Build history of the part. All positions in model axes, mm. A direction names the side the tool comes from. Give positions to 0.01 mm unless a question says otherwise; leave off trailing zeros. Write each loop counter-clockwise with the first axis right and the second up, starting at its lowest first coordinate (ties: lowest second). Pieces come first, ordered by that corner, then holes.
from build123d import *

# Parameters (mm, degrees)
SKETCH_1_W           = 85
SKETCH_1_H           = 65
EXTRUDE_1_DEPTH      = 10
CUT_EXTRUDE_1_REACH  = 109.471
SKETCH_2_R           = 1.7
CUT_EXTRUDE_2_REACH  = 109.471
SKETCH_3_W           = 85
SKETCH_3_H           = 65
CUT_EXTRUDE_4_REACH  = 102.464
CUT_EXTRUDE_7_DEPTH  = 6
SKETCH_6_W           = 4
SKETCH_6_H           = 16
CUT_EXTRUDE_8_DEPTH  = 6
CUT_EXTRUDE_11_DEPTH = 2
SKETCH_15_W          = 14
SKETCH_15_H          = 4.4
CUT_EXTRUDE_13_DEPTH = 8
CHAMFER_1_SIZE       = 1


with BuildPart() as part:
    # 草图1 → 凸台-拉伸1 (new body)
    with BuildSketch(Plane.XY):
        with Locations((42.5, 32.5)):
            Rectangle(SKETCH_1_W, SKETCH_1_H)
    extrude(amount=EXTRUDE_1_DEPTH)

    # 草图2 → 切除-拉伸1 (cut, up to next)
    with BuildSketch(Plane(origin=(0, 0, 0), x_dir=(-1, 0, 0), z_dir=(0, 0, -1)), mode=Mode.PRIVATE) as cut_extrude_1_sk1:
        with Locations((-76.166921514, 56.442524765)):
            Circle(SKETCH_2_R)
    cut_extrude_1_tool1 = extrude(cut_extrude_1_sk1.sketch, amount=-CUT_EXTRUDE_1_REACH, mode=Mode.PRIVATE) & part.part
    # 草图2 → 切除-拉伸1 (cut, up to next)
    with BuildSketch(Plane(origin=(0, 0, 0), x_dir=(-1, 0, 0), z_dir=(0, 0, -1)), mode=Mode.PRIVATE) as cut_extrude_1_sk2:
        with Locations((-8.888803658, 56.442524765)):
            Circle(SKETCH_2_R)
    cut_extrude_1_tool2 = extrude(cut_extrude_1_sk2.sketch, amount=-CUT_EXTRUDE_1_REACH, mode=Mode.PRIVATE) & part.part
    # 草图2 → 切除-拉伸1 (cut, up to next)
    with BuildSketch(Plane(origin=(0, 0, 0), x_dir=(-1, 0, 0), z_dir=(0, 0, -1)), mode=Mode.PRIVATE) as cut_extrude_1_sk3:
        with Locations((-76.166921514, 8.41508509)):
            Circle(SKETCH_2_R)
    cut_extrude_1_tool3 = extrude(cut_extrude_1_sk3.sketch, amount=-CUT_EXTRUDE_1_REACH, mode=Mode.PRIVATE) & part.part
    # 草图2 → 切除-拉伸1 (cut, up to next)
    with BuildSketch(Plane(origin=(0, 0, 0), x_dir=(-1, 0, 0), z_dir=(0, 0, -1)), mode=Mode.PRIVATE) as cut_extrude_1_sk4:
        with Locations((-8.888803658, 8.41508509)):
            Circle(SKETCH_2_R)
    cut_extrude_1_tool4 = extrude(cut_extrude_1_sk4.sketch, amount=-CUT_EXTRUDE_1_REACH, mode=Mode.PRIVATE) & part.part
    add(cut_extrude_1_tool1.solids().sort_by_distance((76.166922, 56.442525, 0))[0], mode=Mode.SUBTRACT)
    add(cut_extrude_1_tool2.solids().sort_by_distance((8.888804, 56.442525, 0))[0], mode=Mode.SUBTRACT)
    add(cut_extrude_1_tool3.solids().sort_by_distance((76.166922, 8.415085, 0))[0], mode=Mode.SUBTRACT)
    add(cut_extrude_1_tool4.solids().sort_by_distance((8.888804, 8.415085, 0))[0], mode=Mode.SUBTRACT)

    # 草图3 → 切除-拉伸2 (cut, up to next)
    with BuildSketch(Plane(origin=(0, 0, 0), x_dir=(-1, 0, 0), z_dir=(0, 0, -1)), mode=Mode.PRIVATE) as cut_extrude_2_sk1:
        with Locations((-42.5, 32.5)):
            Rectangle(SKETCH_3_W, SKETCH_3_H)
        Polygon((-5, 33.462892894), (-5.871324699, 34.334217592), (-5.87504445, 53.137061214), (-5, 54.017366187), (-5, 57.982143592), (-6.992565577, 59.974709169), (-23.773560915, 59.974709169), (-24.394872914, 59.353397171), (-54.61482093, 59.349677419), (-55.245113202, 59.974709169), (-77.982184232, 59.974709169), (-79.974749809, 57.982143592), (-79.97474981, 54.295829484), (-78.032030648, 52.353110322), (-78.028310897, 12.45999492), (-79.97474981, 10.508295484), (-79.97474981, 6.992565577), (-77.982184232, 5), (-74.414239441, 5), (-73.152434681, 6.26180476), (-60.043505207, 6.265524511), (-58.772720173, 5), (-32.926479725, 5), (-31.743585303, 6.182894422), (-17.461559563, 6.186614173), (-16.269684867, 5), (-6.992565577, 5), (-5, 6.992565577), align=None, mode=Mode.SUBTRACT)
    cut_extrude_2_tool1 = extrude(cut_extrude_2_sk1.sketch, amount=-CUT_EXTRUDE_2_REACH, mode=Mode.PRIVATE) & part.part
    add(cut_extrude_2_tool1.solids().sort_by_distance((42.5, 63.929953, 0))[0], mode=Mode.SUBTRACT)

    # 草图4 → 切除-拉伸4 (cut, up to next)
    with BuildSketch(Plane(origin=(0, 0, 0), x_dir=(-1, 0, 0), z_dir=(0, 0, -1)), mode=Mode.PRIVATE) as cut_extrude_4_sk1:
        Polygon((-73.152434681, 6.26180476), (-73.152434681, 20.032317315), (-69.831576581, 23.353175415), (-46.787984184, 23.353175415), (-20.851296271, 23.353175415), (-17.461559563, 19.963438707), (-17.461559563, 6.186614173), (-17.461559563, 0.193960815), (-73.152434681, 0.193960815), align=None)
    cut_extrude_4_tool1 = extrude(cut_extrude_4_sk1.sketch, amount=-CUT_EXTRUDE_4_REACH, mode=Mode.PRIVATE) & part.part
    add(cut_extrude_4_tool1.solids().sort_by_distance((45.311727, 11.681443, 0))[0], mode=Mode.SUBTRACT)

    # 草图5 → 切除-拉伸7 (cut)
    with BuildSketch(Plane(origin=(0, 0, 0), x_dir=(-1, 0, 0), z_dir=(0, 0, -1))):
        Polygon((-24.394872914, 59.353397171), (-24.394872914, 53.906418167), (-25.526104495, 52.774908066), (-53.482640788, 52.774908066), (-54.614150889, 53.906139647), (-54.61482093, 59.349677419), align=None)
    extrude(amount=-CUT_EXTRUDE_7_DEPTH, mode=Mode.SUBTRACT)

    # 草图6 → 切除-拉伸8 (cut)
    with BuildSketch(Plane(origin=(0, 0, 0), x_dir=(-1, 0, 0), z_dir=(0, 0, -1))):
        with Locations((-7.871324699, 42.334217592)):
            Rectangle(SKETCH_6_W, SKETCH_6_H)
    extrude(amount=-CUT_EXTRUDE_8_DEPTH, mode=Mode.SUBTRACT)

    # 草图7 → 切除-拉伸11 (cut)
    with BuildSketch(Plane(origin=(0, 0, 0), x_dir=(-1, 0, 0), z_dir=(0, 0, -1))):
        Polygon((-74.432117646, 51.26230094), (-76.432117646, 51.26230094), (-78.031928938, 51.26230094), (-78.029847328, 28.93771831), (-75.029847328, 28.93771831), (-75.029847328, 13.93771831), (-73.152434681, 12.060305663), (-73.152434681, 20.032317315), (-69.831576581, 23.353175415), (-20.851296271, 23.353175415), (-17.461559563, 19.963438707), (-17.461559563, 6.186614173), (-16.269684867, 5), (-12.014024847, 5), (-12.014024847, 10.599811284), (-10.599811284, 12.014024847), (-6.599811284, 12.014024847), (-5, 12.014024847), (-5, 33.462892894), (-5.871324699, 34.334217592), (-9.871324699, 34.334217592), (-9.871324699, 50.334217592), (-5.874489966, 50.334217592), (-5.87504445, 53.137061214), (-9.87504445, 53.137061214), (-12.071959353, 55.333976117), (-12.071959353, 58.333976117), (-12.071959353, 59.974709169), (-23.773560915, 59.974709169), (-24.394872914, 59.353397171), (-24.394872914, 53.906418167), (-25.526104495, 52.774908066), (-53.482640788, 52.774908066), (-54.614150889, 53.906139647), (-54.61482093, 59.349677419), (-55.245113202, 59.974709169), (-71.319520701, 59.974709169), (-71.319520701, 58.374897885), (-71.319520701, 54.374897885), align=None)
    extrude(amount=-CUT_EXTRUDE_11_DEPTH, mode=Mode.SUBTRACT)

    # 草图15 → 切除-拉伸13 (cut)
    with BuildSketch(Plane.XY.offset(10)):
        with Locations((48.428848604, 25.553175415)):
            Rectangle(SKETCH_15_W, SKETCH_15_H)
    extrude(amount=-CUT_EXTRUDE_13_DEPTH, mode=Mode.SUBTRACT)

    # 倒角1
    chamfer_1_edges = [part.edges().sort_by_distance(p)[0] for p in [
        (55.428848604, 23.353175415, 6),
        (55.428848604, 27.753175415, 6),
        (41.428848604, 27.753175415, 6),
        (41.428848604, 23.353175415, 6),
    ]]
    chamfer(chamfer_1_edges, length=CHAMFER_1_SIZE)


solid = part.part
1. Drop flat-ended pins along their axis: pin 1 (7 mm diameter, centred on x = 42.5, y = 57.5, fed in from -Z); pin 2 (2 mm diameter, centred on x = 51, z = 7.5, fed in from -Y); pin 3 (4 mm diameter, centred on y = 19, z = 5.5, fed in from +X); pin 4 (2 mm diameter, centred on x = 8.89, y = 56.44, fed in from -Z). Give the stop position or say it passes through.
2. Mould opens along Y. For faces 5 (the face through (39, 56, 6)), 6 (the face through (12, 5, 5)), 7 (the face through (8, 53.137, 1)) say: pulls with the +Y half, pulls with the -Y half, needs draft (parallel to the pull), parting line crosses it, or undercut.
3. 3-axis set-ups, long thin cutter, end or side, ignore diameter. For faces 1 (the face through (8, 12.014, 1)), 2 (the face through (39, 52.775, 4)), 3 (the face through (71.515, 21.67, 5.944)), 4 (the face through (76, 51.262, 1)): which of +Z, -Z, +X, -X, +Y, -Y reach the whole face in a straight line?
4. Drill centre lines: line 1 along X through (y, z) = (8.5, 3.25); line 2 along Y through (x, z) = (8.5, 3.25); line 3 along Z through (x, y) = (52, 32.5). Where is each one in solid material? Low to high.
5. Saw through at D-D on x = 62.5. Give the cut face in (y, z).
6. Saw through at A-A on x = 52. Give the cut face in (y, z).
7. Saw through at B-B on y = 30.5. Give the cut face in (x, z).
8. Saw through at C-C on z = 4. Count the separate pieces of the cut face and the enclosed holes in it, plus the area to 3 significant figures.
Outcome:
1. pin 1: stops at z = 6
1. pin 2: stops at y = 27.75
1. pin 3: stops at x = 78.03
1. pin 4: passes through
2. face 5: needs draft
2. face 6: pulls with the -Y half
2. face 7: undercut
3. face 1: -Z, -X
3. face 2: -Z, +Y
3. face 3: +Z, -Z, -Y
3. face 4: -Z, +X, -X
4. line 1: x = 5 to 7.19, 10.59 to 17.46, 73.15 to 74.47, 77.86 to 79.97
4. line 2: y = 5 to 6.76, 10.07 to 34.33, 50.33 to 54.79, 58.1 to 59.97
4. line 3: z = 2 to 10
5. outline: (23.35, 2) - (59.97, 2) - (59.97, 10) - (23.35, 10) - close
6. outline: (27.75, 2) - (52.77, 2) - (52.77, 6) - (59.35, 6) - (59.35, 10) - (27.75, 10) - close
7. outline: (5, 2) - (78.03, 2) - (78.03, 10) - (5, 10) - close
8. separate pieces: 1
8. enclosed holes: 4
8. area: 2,620 mm2
